Verification items for the finished model (mm, model axes). A direction names the side the tool comes from. Coordinates: 2 decimals unless noted, no trailing zeros. Write each loop counter-clockwise with the first axis right and the second up, starting at its lowest first coordinate (ties: lowest second). Pieces come first, ordered by that corner, then holes. Notation, with made-up numbers: (-2.5, 72) -> (37.5, 72) arc R27 ccw to (37.5, 95) -> close; hole circle Ø7 at (86.25, 72). An arc over 180 degrees is marked (long way). Answer in a Markdown table with one row per item.
```python
from build123d import *

# Parameters (mm, degrees)
F0_W        = 43
F0_H        = 22
F1_DEPTH    = 53
F2_T        = -3
F3_W        = 37
F3_H        = 0.5
F4_DEPTH    = 1
F5_R        = 0.49999
F6_R        = 2
F7_T1_DEPTH = 37


# Not quite as in the source:
# - a fillet or chamfer that OpenCascade refuses, or shapes differently, is made with other operations: its cross-section is extruded or revolved along the edge and cut away or added
# - a fillet or chamfer is up to 0.001 mm smaller than in the source, because OpenCascade refuses the exact size


with BuildPart() as f1:
    # F0 (on Top) → F1 (new body)
    with BuildSketch(Plane.XY):
        Rectangle(F0_W, F0_H)
    extrude(amount=F1_DEPTH)

    # F2
    f2_openings = [f1.faces().sort_by_distance(p)[0] for p in [
        (0, 0, 53),
    ]]
    offset(amount=F2_T, openings=f2_openings)

    # F3 (on face) → F4 (join)
    with BuildSketch(Plane.XY.offset(53)):
        with Locations((0, 7.75)):
            Rectangle(F3_W, F3_H)
    extrude(amount=-F4_DEPTH)

    # F5 (radius 0.5 in the source; OpenCascade refuses exactly that, so slightly less here)
    f5_edges = [f1.edges().sort_by_distance(p)[0] for p in [
        (0, 7.5, 53),
        (0, 7.5, 52),
    ]]
    fillet(f5_edges, radius=F5_R)

    # F6
    f6_edges = [f1.edges().sort_by_distance(p)[0] for p in [
        (21.5, -11, 26.5),
        (-21.5, -11, 26.5),
        (21.5, 0, 0),
        (0, 11, 0),
        (-21.5, 0, 0),
        (0, -11, 0),
        (-21.5, 0, 53),
        (0, 11, 53),
        (21.5, 0, 53),
        (0, -11, 53),
    ]]
    fillet(f6_edges, radius=F6_R)

    # F7: fillet of radius 7 on 1 edges, made by hand

    # F7_s2 → F7_t1 (cut)
    with BuildSketch(Plane.YZ.offset(-18.5)):
        with BuildLine():
            ThreePointArc((-15, 53), (-10.0502525317, 50.9497474683), (-8, 46))
            Line((-8, 46), (-7.86, 46))
            Line((-7.86, 46), (-7.86, 53.14))
            Line((-7.86, 53.14), (-15, 53.14))
            Line((-15, 53.14), (-15, 53))
        make_face()
    extrude(amount=F7_T1_DEPTH, mode=Mode.SUBTRACT)


solid = f1.part
```
1. Sectioned sample at B-B, the plane y = 6. Record the cut outline in (x, z), and give its area (3 significant figures).
Findings below:
| item | result |
|---|---|
| outline | (-21.5, 2) arc R2 ccw to (-19.5, 0) -> (19.5, 0) arc R2 ccw to (21.5, 2) -> (21.5, 51) arc R2 ccw to (19.5, 53) -> (18.5, 53) -> (18.5, 3) -> (-18.5, 3) -> (-18.5, 53) -> (-19.5, 53) arc R2 ccw to (-21.5, 51) -> close |
| area | 426 mm² |
2. Release check for a two-part mould opening along X. For faces 3 (the face through (-20.9, 1.14, 52.43)), 4 (the face through (0, 11, 26)), 5 (the face through (-0.259, -8.784, 49.22)) record: released by +X, released by -X, zero draft, split by the parting line, or undercut.
Findings below:
| item | result |
|---|---|
| face 3 | released by -X |
| face 4 | zero draft |
| face 5 | undercut |
3. Go/stop test with a flat-tipped pin: pin 1 (13 mm diameter, centred on x = -1.5, y = -2.5, fed in from +Z). Record where the tip stops, or that it passes through.
Findings below:
| item | result |
|---|---|
| pin 1 | stops at z = 49.61 |
4. Material ranges on probe 1 along Y at (x, z) = (-5.5, 38.5); probe 2 along X at (y, z) = (5, 42.5); probe 3 along Z at (x, y) = (0, 7.25), recorded low to high. Write a range as from..to.
Findings below:
| item | result |
|---|---|
| probe 1 | y = -11..-8, 8..11 |
| probe 2 | x = -21.5..-18.5, 18.5..21.5 |
| probe 3 | z = 0..3 |
5. Sectioned sample at C-C, the plane z = 8. Record the cut outline in (x, y).
Findings below:
| item | result |
|---|---|
| outline | (-21.5, -9) arc R2 ccw to (-19.5, -11) -> (19.5, -11) arc R2 ccw to (21.5, -9) -> (21.5, 11) -> (-21.5, 11) -> close; hole (-18.5, -8) -> (18.5, -8) -> (18.5, 8) -> (-18.5, 8) -> close |
6. Access from +Z, -Z, +X, -X, +Y, -Y to the whole of each face (thin tool, end or side, straight path). Record for faces 1 (the face through (0, -8, 24)), 2 (the face through (20.9, 1.14, 0.57)).
Findings below:
| item | result |
|---|---|
| face 1 | +Z |
| face 2 | -Z, +X, +Y, -Y |
